```python
from build123d import *

# Parameters (mm, degrees)
SKETCH1_W           = 11.5
SKETCH1_H           = 5.5
BOSS_EXTRUDE1_DEPTH = 2
SKETCH3_W           = 2
SKETCH3_H           = 2
BOSS_EXTRUDE2_DEPTH = 2
SKETCH5_W           = 0.6
SKETCH5_H           = 0.25
BOSS_EXTRUDE3_DEPTH = 2


with BuildPart() as part:
    # Sketch1 → Boss-Extrude1 (new, symmetric)
    with BuildSketch(Plane(origin=(0, 0, 0), x_dir=(1, 0, 0), z_dir=(0, 1, 0))):
        Rectangle(SKETCH1_W, SKETCH1_H)
    extrude(amount=BOSS_EXTRUDE1_DEPTH, both=True)

    # Sketch3 → Boss-Extrude2 (add)
    with BuildSketch(Plane.XY.offset(2.75)):
        with Locations((-1.5, 0)):
            Rectangle(SKETCH3_W, SKETCH3_H)
    extrude(amount=BOSS_EXTRUDE2_DEPTH)

    # Sketch5 → Boss-Extrude3 (add)
    with BuildSketch(Plane(origin=(0, 0, -2.75), x_dir=(-1, 0, 0), z_dir=(0, 0, -1))):
        with Locations((-2.54, 0)):
            Rectangle(SKETCH5_W, SKETCH5_H)
        Rectangle(SKETCH5_W, SKETCH5_H)
        with Locations((2.54, 0)):
            Rectangle(SKETCH5_W, SKETCH5_H)
    extrude(amount=BOSS_EXTRUDE3_DEPTH)


solid = part.part
```
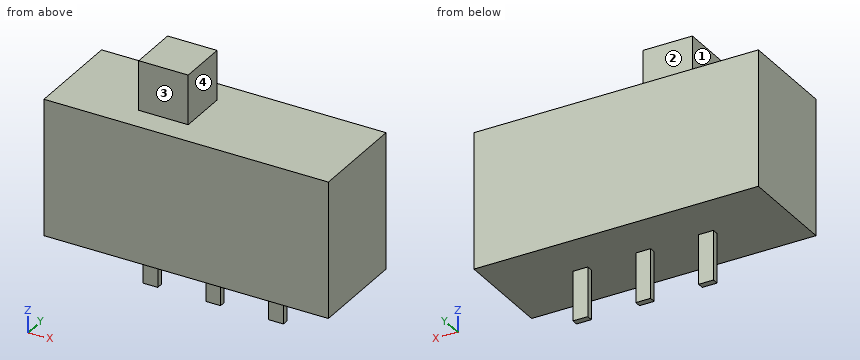
Work out the finished part from the listing and answer in its coordinate system (mm). Face numbers are marked on the shaded views. A direction names the side the tool comes from. Give positions to 0.01 mm unless a question says otherwise; leave off trailing zeros. Loops run counter-clockwise (first coordinate to the right, second up) from the corner with the lowest first, then second, coordinate; pieces in that order, holes last. Notation, with made-up numbers: (18, -12) -> (66, -12) arc R5 cw to (66, -4) -> close; hole circle Ø6 at (26, 87). An arc over 180 degrees is marked (long way). Put each result on its own line as item: value. Start each with the question number.
Item 1: Which of the six approach directions +Z, -Z, +X, -X, +Y, -Y give full straight-line access (tool end or side, diameter ignored) to the marked faces 1, 2, 3 and 4?
Item 2: The part is cut by section C-C (y = 0.55). Give the vertices of the cut face in (x, z), then the cut area to 4 significant figures.
Item 3: The part is cut by section B-B (x = -1). Give the vertices of the cut face in (y, z).
Item 4: The part is cut by section A-A (z = -3.75). Give the vertices of the cut face in (x, y) (3 decimals).
Item 5: Each of these flat-tipped pins is pushed along its axis until it touches: P1, Ø1.5, axis at x = 1.5, y = -1, coming from the -Z side; P2, Ø2, axis at x = -1.5, z = 4, coming from the -Y side; P3, Ø2, axis at x = 3.5, y = 0.5, coming from the -Z side; P4, Ø2, axis at x = -2, z = 4, coming from the +Y side. Where does it stop, or does it pass through?
Item 6: The part is cut by section D-D (z = 4). Give the vertices of the cut face in (x, y).
Item 7: Find the intervals of material crossed by L1, parallel to Z at x = -1.75, y = -0.3; L2, parallel to Z at x = 0.5, y = -1.65; L3, parallel to X at y = -0.85, z = 4.25, in increasing order. Write a range as [from, to].
Answers below:
1. face 1: +Z, -X, +Y, -Y
1. face 2: +Z, +X, -X, +Y
1. face 3: +Z, +X, -X, -Y
1. face 4: +Z, +X, +Y, -Y
2. outline: (-5.75, -2.75) -> (5.75, -2.75) -> (5.75, 2.75) -> (-0.5, 2.75) -> (-0.5, 4.75) -> (-2.5, 4.75) -> (-2.5, 2.75) -> (-5.75, 2.75) -> close
2. area: 67.25 mm2
3. outline: (-2, -2.75) -> (2, -2.75) -> (2, 2.75) -> (1, 2.75) -> (1, 4.75) -> (-1, 4.75) -> (-1, 2.75) -> (-2, 2.75) -> close
4. outline: (-2.84, -0.125) -> (-2.24, -0.125) -> (-2.24, 0.125) -> (-2.84, 0.125) -> close; (-0.3, -0.125) -> (0.3, -0.125) -> (0.3, 0.125) -> (-0.3, 0.125) -> close; (2.24, -0.125) -> (2.84, -0.125) -> (2.84, 0.125) -> (2.24, 0.125) -> close
5. P1: z = -2.75
5. P2: y = -1
5. P3: z = -4.75
5. P4: y = 1
6. outline: (-2.5, -1) -> (-0.5, -1) -> (-0.5, 1) -> (-2.5, 1) -> close
7. L1: [-2.75, 4.75]
7. L2: [-2.75, 2.75]
7. L3: [-2.5, -0.5]
